Study the drawing (mm; zero at the part's minimum x, y, z) and answer. Coordinates: 2 decimals unless noted, no trailing zeros. Order: outer loops, then holes, each group sorted by start corner. A loop starts at its lowest first (then second) coordinate and runs counter-clockwise, first axis right, second up. Notation, with made-up numbers: (-7, -18) -> (21, -18) arc R13 ccw to (21, -5) -> close; hole circle Ø7 at (77, 61). An arc over 180 degrees is marked (long way). Write each question's results on one line, items separated by ' | '. Start each with the question number.
(1) Straight lines are drawn through the part: L1, parallel to Y at x = 24.5, z = 3.5; L2, parallel to X at y = 15.5, z = 6.5; L3, parallel to Y at x = 40, z = 5.25 (1 decimal). For each, find the intervals that lie inside material, in ascending order.
(2) The part is cut by section A-A, the plane z = 6.75. Give the vertices of the cut face in (x, y) (1 decimal), then the cut area to 3 significant figures.
(3) Given pin 1 (1 mm diameter, centred on y = 29.5, z = 4, fed in from -X) (1 decimal); pin 2 (4 mm diameter, centred on x = 24.5, y = 7.3, fed in from +Z); pin 3 (3 mm diameter, centred on x = 30.5, z = 6, fed in from +Y) (1 decimal); pin 4 (2 mm diameter, centred on y = 5.5, z = 6, fed in from +X), each flat-ended and moving along its own axis, determine where each tip first touches the part or whether it passes through.
(4) The part is cut by section B-B, the plane x = 24.5. Give the vertices of the cut face in (y, z), then the cut area to 3 significant figures.
(5) Determine the mould class of the marked faces 1, 2, 3 and 4 for opening direction Y: +Y half, -Y half, draft (parallel to the pull), parting line (faces both ways), or undercut.
(6) The part is cut by section C-C, the plane y = 15.9. Give the vertices of the cut face in (x, z) (1 decimal).
(7) The part is cut by section D-D, the plane y = 24.5. Give the vertices of the cut face in (x, z).
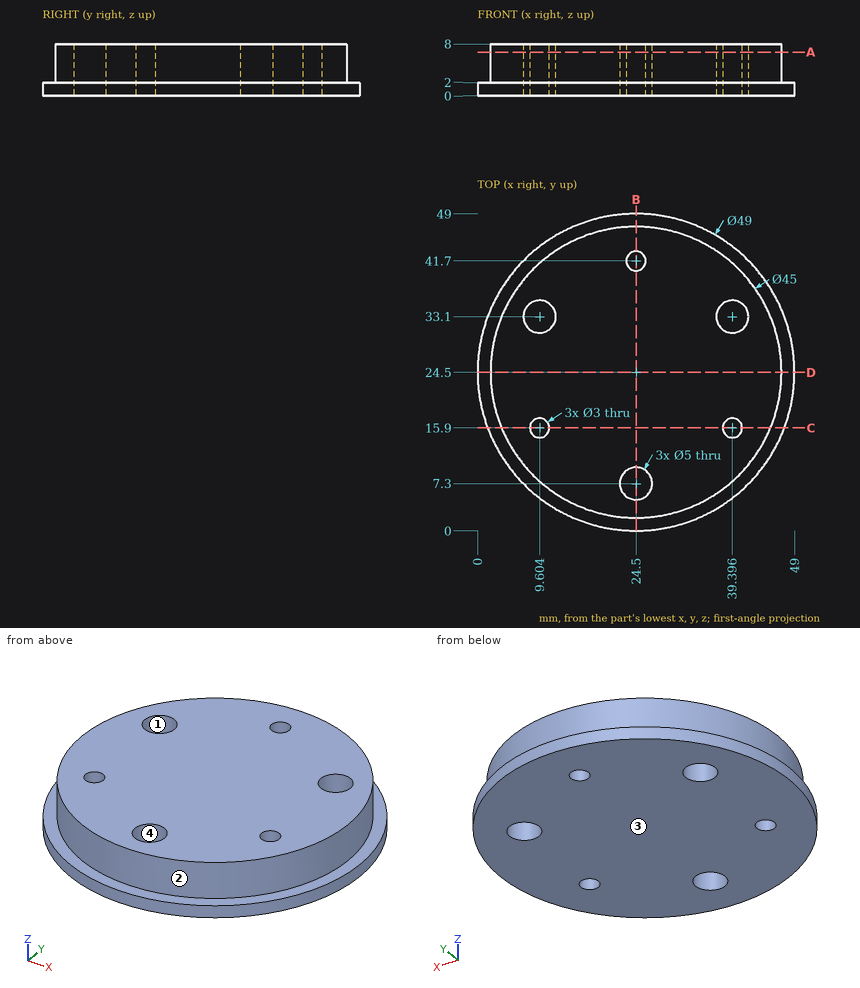
Established:
1) L1: y = 2 to 4.8, 9.8 to 40.2, 43.2 to 47 | L2: x = 3.88 to 8.16, 11.05 to 37.95, 40.84 to 45.12 | L3: y = 8.2 to 14.5, 17.3 to 30.7, 35.5 to 40.8
2) outline: circle Ø45 at (24.5, 24.5); hole circle Ø5 at (9.6, 33.1); hole circle Ø3 at (9.6, 15.9); hole circle Ø5 at (24.5, 7.3); hole circle Ø3 at (24.5, 41.7); hole circle Ø5 at (39.4, 33.1); hole circle Ø3 at (39.4, 15.9) | area: 1,510 mm^2
3) pin 1: stops at x = 2.5 | pin 2: passes through | pin 3: stops at y = 46.5 | pin 4: stops at x = 38
4) outline: (0, 0) -> (4.8, 0) -> (4.8, 8) -> (2, 8) -> (2, 2) -> (0, 2) -> close; (9.8, 0) -> (40.2, 0) -> (40.2, 8) -> (9.8, 8) -> close; (43.2, 0) -> (49, 0) -> (49, 2) -> (47, 2) -> (47, 8) -> (43.2, 8) -> close | area: 304 mm^2
5) face 1: undercut | face 2: parting line | face 3: draft | face 4: undercut
6) outline: (1.6, 0) -> (8.1, 0) -> (8.1, 8) -> (3.7, 8) -> (3.7, 2) -> (1.6, 2) -> close; (11.1, 0) -> (37.9, 0) -> (37.9, 8) -> (11.1, 8) -> close; (40.9, 0) -> (47.4, 0) -> (47.4, 2) -> (45.3, 2) -> (45.3, 8) -> (40.9, 8) -> close
7) outline: (0, 0) -> (49, 0) -> (49, 2) -> (47, 2) -> (47, 8) -> (2, 8) -> (2, 2) -> (0, 2) -> close
